The model under review builds one solid part; all positions refer to its coordinate system, in mm. A direction names the side the tool comes from. Coordinates: 2 decimals unless noted, no trailing zeros. Loops run counter-clockwise (first coordinate to the right, second up) from the corner with the lowest first, then second, coordinate; pieces in that order, holes last. Notation, with made-up numbers: (85, 6) - (94, 6) arc R27 ccw to (94, 40) - close; hole circle Ø6 at (37.5, 76.5). An arc over 180 degrees is marked (long way). Use a Markdown table: item, result. Add a question column.
1) To check wall thickness, follow L1, parallel to X at y = 5, z = 1; L2, parallel to X at y = 2, z = 1.75; L3, parallel to Y at x = 1, z = 7.5. State the ranges of each line that lie inside material, in increasing order. Write a range as [from, to].
2) Add section B-B, the plane z = 4.25. Give the boundary of the cut face in (x, y), and give its area (3 significant figures).
3) Add section D-D, the plane x = 9.5. Give the boundary of the cut face in (y, z).
4) Clearance check with flat-ended pins moving along their axes: pin 1 (1.2 mm diameter, centred on x = -8.5, y = 2, fed in from -Z); pin 2 (5 mm diameter, centred on x = 9, z = 9.5, fed in from +Y); pin 3 (3.5 mm diameter, centred on x = -11.5, y = 1.5, fed in from +Z); pin 4 (3 mm diameter, centred on y = 6.5, z = 3, fed in from +X). State where each tip first meets the part, or that it passes through.
5) For faces 1 (the flat face through (-10.4, 3, 4.2)), 2 (the flat face through (-8, 1, 3.05)), 3 (the flat face through (-5.813, 4, 6)), 4 (the flat face through (10.4, 3, 4.2)), list the 3-axis set-ups (+Z, -Z, +X, -X, +Y, -Y) from which the entire face can be reached by the end or side of a thin tool; tool diameter is ignored.
6) Add section C-C, the plane z = 1.5. Give the boundary of the cut face in (x, y), and give its area (3 significant figures).
7) Add section A-A, the plane y = 2.5. Give the boundary of the cut face in (x, z), and give its area (3 significant figures).
8) The part is to be moulded in two halves that separate along X. For faces 5 (the cylindrical face through (-7.05, 11.07, 5.83)), 6 (the flat face through (10, 1, 8.5)), 7 (the cylindrical face through (-5.361, 9.572, 5.83)), say which applies: pulls with the +X half, pulls with the -X half, needs draft (parallel to the pull), parting line crosses it, or undercut.
```python
from build123d import *

# Parameters (mm, degrees)
EXTRUDE_1_DEPTH     = 11.5
SKETCH_3_W          = 11.812534662
SKETCH_3_H          = 10
CUT_EXTRUDE_1_DEPTH = 11.5
FILLET_1_R          = 1.5
FILLET_2_R          = 1.5
FILLET_3_R          = 1.5
FILLET_4_R          = 1.5
SKETCH_5_W          = 5.8
SKETCH_5_H          = 8.5
EXTRUDE_2_DEPTH     = 3
HOLE_WIZARD_M2_1_D  = 2.4
SKETCH_9_W          = 1.5
SKETCH_9_H          = 2.4
CUT_EXTRUDE_4_DEPTH = 3


with BuildPart() as part:
    # ｽｹｯﾁ1 → ﾎﾞｽ - 押し出し1 (new body)
    with BuildSketch(Plane.XY):
        Polygon((0, 0), (7.5, 0), (7.5, 11.5), (-7.5, 11.5), (-7.5, 0), align=None)
    extrude(amount=EXTRUDE_1_DEPTH)

    # ｽｹｯﾁ3 → ｶｯﾄ - 押し出し1 (cut)
    with BuildSketch(Plane.XY):
        with Locations((0.093732669, 5)):
            Rectangle(SKETCH_3_W, SKETCH_3_H)
    extrude(amount=CUT_EXTRUDE_1_DEPTH, mode=Mode.SUBTRACT)

    # ﾌｨﾚｯﾄ1
    fillet_1_edges = [part.edges().sort_by_distance(p)[0] for p in [
        (6, 10, 5.75),
    ]]
    fillet(fillet_1_edges, radius=FILLET_1_R)

    # ﾌｨﾚｯﾄ2
    fillet_2_edges = [part.edges().sort_by_distance(p)[0] for p in [
        (-5.812534662, 10, 5.75),
    ]]
    fillet(fillet_2_edges, radius=FILLET_2_R)

    # ﾌｨﾚｯﾄ3
    fillet_3_edges = [part.edges().sort_by_distance(p)[0] for p in [
        (7.5, 11.5, 5.75),
    ]]
    fillet(fillet_3_edges, radius=FILLET_3_R)

    # ﾌｨﾚｯﾄ4
    fillet_4_edges = [part.edges().sort_by_distance(p)[0] for p in [
        (-7.5, 11.5, 5.75),
    ]]
    fillet(fillet_4_edges, radius=FILLET_4_R)

    # ｽｹｯﾁ5 → ﾎﾞｽ - 押し出し2 (add)
    with BuildSketch(Plane(origin=(0, 0, 0), x_dir=(1, 0, 0), z_dir=(0, 1, 0))):
        with Locations((-10.4, -4.25)):
            Rectangle(SKETCH_5_W, SKETCH_5_H)
        with Locations((10.4, -4.25)):
            Rectangle(SKETCH_5_W, SKETCH_5_H)
    extrude(amount=EXTRUDE_2_DEPTH)

    # M2 すきま穴1 (through all)
    with Locations(Plane(origin=(0, 0, 0), x_dir=(-1, 0, 0), z_dir=(0, -1, 0))):
        with Locations((9, -4.25), (-9, -4.25)):
            Hole(HOLE_WIZARD_M2_1_D / 2)

    # ｽｹｯﾁ9 → ｶｯﾄ - 押し出し4 (cut)
    with BuildSketch(Plane(origin=(0, 0, 0), x_dir=(1, 0, 0), z_dir=(0, 1, 0))):
        with Locations((8.25, -4.25)):
            Rectangle(SKETCH_9_W, SKETCH_9_H)
        with Locations((-8.25, -4.25)):
            Rectangle(SKETCH_9_W, SKETCH_9_H)
    extrude(amount=CUT_EXTRUDE_4_DEPTH, mode=Mode.SUBTRACT)


solid = part.part
```
From the geometry:
| question | item | result |
|---|---|---|
| 1 | L1 | x = [-7.5, -5.81], [6, 7.5] |
| 1 | L2 | x = [-13.3, -5.81], [6, 13.3] |
| 1 | L3 | y = [10, 11.5] |
| 2 | outline | (-13.3, 0) - (-10.2, 0) - (-10.2, 3) - (-13.3, 3) - close; (-7.5, 0) - (-5.81, 0) - (-5.81, 8.5) arc R1.5 cw to (-4.31, 10) - (4.5, 10) arc R1.5 cw to (6, 8.5) - (6, 0) - (7.5, 0) - (7.5, 10) arc R1.5 ccw to (6, 11.5) - (-6, 11.5) arc R1.5 ccw to (-7.5, 10) - close; (10.2, 0) - (13.3, 0) - (13.3, 3) - (10.2, 3) - close |
| 2 | area | 73.0 mm^2 |
| 3 | outline | (0, 0) - (3, 0) - (3, 3.16) - (0, 3.16) - close; (0, 5.34) - (3, 5.34) - (3, 8.5) - (0, 8.5) - close |
| 4 | pin 1 | stops at z = 0 |
| 4 | pin 2 | stops at y = 11.41 |
| 4 | pin 3 | stops at z = 8.5 |
| 4 | pin 4 | stops at x = 7.5 |
| 5 | face 1 | +Z, -Z, -X, +Y |
| 5 | face 2 | +Y, -Y |
| 5 | face 3 | +Z, -Z, -Y |
| 5 | face 4 | +Z, -Z, +X, +Y |
| 6 | outline | (-13.3, 0) - (-5.81, 0) - (-5.81, 8.5) arc R1.5 cw to (-4.31, 10) - (4.5, 10) arc R1.5 cw to (6, 8.5) - (6, 0) - (13.3, 0) - (13.3, 3) - (7.5, 3) - (7.5, 10) arc R1.5 ccw to (6, 11.5) - (-6, 11.5) arc R1.5 ccw to (-7.5, 10) - (-7.5, 3) - (-13.3, 3) - close |
| 6 | area | 89.2 mm^2 |
| 7 | outline | (-13.3, 0) - (-5.81, 0) - (-5.81, 11.5) - (-7.5, 11.5) - (-7.5, 8.5) - (-13.3, 8.5) - close; (6, 0) - (13.3, 0) - (13.3, 8.5) - (7.5, 8.5) - (7.5, 11.5) - (6, 11.5) - close; hole (-9, 3.05) - (-7.5, 3.05) - (-7.5, 5.45) - (-9, 5.45) arc R1.2 ccw to start; hole (7.5, 3.05) - (9, 3.05) arc R1.2 ccw to (9, 5.45) - (7.5, 5.45) - close |
| 7 | area | 124 mm^2 |
| 8 | face 5 | pulls with the -X half |
| 8 | face 6 | needs draft |
| 8 | face 7 | undercut |
